```python
from build123d import *

# Parameters (mm, degrees)
CROQUIS2_R              = 14.5
SALIENTE_EXTRUIR1_DEPTH = 35
CROQUIS3_R              = 2.675
CORTAR_EXTRUIR1_DEPTH   = 14
CROQUIS7_R              = 3
CORTAR_EXTRUIR6_DEPTH   = 4.7
CORTAR_EXTRUIR8_START   = 9.8
CORTAR_EXTRUIR8_DEPTH   = 3
CORTAR_EXTRUIR2_REACH   = 42.565
CROQUIS4_R              = 1.75


with BuildPart() as part:
    # Croquis2 → Saliente-Extruir1 (new, symmetric)
    with BuildSketch(Plane(origin=(0, 0, 0), x_dir=(1, 0, 0), z_dir=(0, 1, 0))):
        with Locations(Location((0, 0, 0), (0, 0, 270))):
            Circle(CROQUIS2_R)
    extrude(amount=SALIENTE_EXTRUIR1_DEPTH, both=True)

    # Croquis3 → Cortar-Extruir1 (cut)
    with BuildSketch(Plane(origin=(0, 35, 0), x_dir=(1, 0, 0), z_dir=(0, 1, 0))):
        with Locations(Location((0, 0, 0), (0, 0, 270))):
            Circle(CROQUIS3_R)
    cortar_extruir1 = extrude(amount=-CORTAR_EXTRUIR1_DEPTH, mode=Mode.SUBTRACT)

    # Croquis7 → Cortar-Extruir6 (cut)
    with BuildSketch(Plane.XY.offset(14.5)):
        with Locations((0, 23)):
            Circle(CROQUIS7_R)
    cortar_extruir6 = extrude(amount=-CORTAR_EXTRUIR6_DEPTH, mode=Mode.SUBTRACT)

    # Croquis5 → Cortar-Extruir8 (cut)
    with BuildSketch(Plane.XY.offset(CORTAR_EXTRUIR8_START)):
        Polygon((-1.5, 20.401923789), (1.5, 20.401923789), (3, 23), (1.5, 25.598076211), (-1.5, 25.598076211), (-3, 23), align=None)
    cortar_extruir8 = extrude(amount=-CORTAR_EXTRUIR8_DEPTH, mode=Mode.SUBTRACT)

    # Croquis4 → Cortar-Extruir2 (cut, up to next)
    with BuildSketch(Plane.XY, mode=Mode.PRIVATE) as cortar_extruir2_sk1:
        with Locations(Location((0, 23, 0), (0, 0, 180))):
            Circle(CROQUIS4_R)
    cortar_extruir2_tool1 = extrude(cortar_extruir2_sk1.sketch, amount=CORTAR_EXTRUIR2_REACH, mode=Mode.PRIVATE) & part.part
    cortar_extruir2 = cortar_extruir2_tool1.solids().sort_by_distance((0, 23, 0))[0]
    add(cortar_extruir2, mode=Mode.SUBTRACT)

    # Simetría2: Cortar-Extruir1, Cortar-Extruir6, Cortar-Extruir8, Cortar-Extruir2 across plane
    add(cortar_extruir1.mirror(Plane.ZX), mode=Mode.SUBTRACT)
    add(cortar_extruir6.mirror(Plane.ZX), mode=Mode.SUBTRACT)
    add(cortar_extruir8.mirror(Plane.ZX), mode=Mode.SUBTRACT)
    add(cortar_extruir2.mirror(Plane.ZX), mode=Mode.SUBTRACT)


solid = part.part
```
Verification items for the finished model (mm, model axes). A direction names the side the tool comes from. Coordinates: 2 decimals unless noted, no trailing zeros. Loops run counter-clockwise (first coordinate to the right, second up) from the corner with the lowest first, then second, coordinate; pieces in that order, holes last. Notation, with made-up numbers: (16, 88) - (26, 88) arc R10 cw to (26, 100) - close; hole circle Ø5 at (74.5, 20.5). An arc over 180 degrees is marked (long way). Put each result on its own line as item: value.
Item 1: Scan lines: line 1 along Y through (x, z) = (0, 13.1); line 2 along X through (y, z) = (25, 0) (3 decimals); line 3 along X through (y, z) = (-23, 4.45). Record each from-to range of solid material in increasing order.
Conclusion:
line 1: y = -35 to -26, -20 to 20, 26 to 35
line 2: x = -14.5 to -2.675, 2.675 to 14.5
line 3: x = -13.8 to -1.75, 1.75 to 13.8
Item 2: Draft check along Y on faces 4 (the face through (0, -21, 0)), 5 (the face through (2.4, 24.4, 9.8)). Enter one of: pulls with the +Y half, pulls with the -Y half, needs draft (parallel to the pull), parting line crosses it, or undercut.
Conclusion:
face 4: pulls with the -Y half
face 5: undercut
Item 3: Set-up check for faces 1 (the face through (-1.669, 22.474, 4.378)), 2 (the face through (0.118, -28.098, -2.672)), 3 (the face through (0.118, 28.098, -2.672)): record each of +Z, -Z, +X, -X, +Y, -Y from which the full face is reachable in a straight line by a thin tool's end or side.
Conclusion:
face 1: +Z
face 2: -Y
face 3: +Y
Item 4: Section check C-C (y = 6.5). Enter the section's corners in (x, z), then the cut area to 3 significant figures.
Conclusion:
outline: circle Ø29 at (0, 0)
area: 661 mm2
Item 5: Section check A-A (z = 0). Enter the section's corners in (x, y) (3 decimals).
Conclusion:
outline: (-14.5, -35) - (-2.675, -35) - (-2.675, -21) - (2.675, -21) - (2.675, -35) - (14.5, -35) - (14.5, 35) - (2.675, 35) - (2.675, 21) - (-2.675, 21) - (-2.675, 35) - (-14.5, 35) - close
Item 6: Section check B-B (y = 28). Enter the section's corners in (x, z) (3 decimals), then the cut area to 3 significant figures.
Conclusion:
outline: circle Ø29 at (0, 0); hole circle Ø5.35 at (0, 0)
area: 638 mm2
Item 7: Gauge pin test, flat ends, axial feed: pin 1 Ø0.8 at (x, y) = (2, 21) entering from +Z; pin 2 Ø0.8 at (x, y) = (-2.5, -23.5) entering from +Z; pin 3 Ø1.5 at (y, z) = (2, 7) entering from -X. Record the tip position at first contact, or that the pin passes through.
Conclusion:
pin 1: stops at z = 14.38
pin 2: stops at z = 9.8
pin 3: stops at x = -13.08
Item 8: Section check D-D (x = 10.75). Enter the section's corners in (y, z), then the cut area to 3 significant figures.
Conclusion:
outline: (-35, -9.73) - (35, -9.73) - (35, 9.73) - (-35, 9.73) - close
area: 1,360 mm2
